Design review of the part shown in the three views and the two pictorial views. Dimensions are in mm from the part's minimum x, y and z. A direction names the side the tool comes from. Coordinates: 2 decimals unless noted, no trailing zeros. Order: outer loops, then holes, each group sorted by start corner. A loop starts at its lowest first (then second) coordinate and runs counter-clockwise, first axis right, second up. Notation, with made-up numbers: (63, -36.75) - (88, -36.75) arc R16 ccw to (88, -31.75) - close; hole circle Ø10 at (23.25, 23.25). An arc over 180 degrees is marked (long way). One line per item, written item: value. Start each with the question number.
(1) To check wall thickness, follow line 1 along Z through (x, y) = (105.5, 37.5); line 2 along X through (y, z) = (26.5, 12); line 3 along Z through (x, y) = (164, 74). State the ranges of each line that lie inside material, in increasing order.
(2) For the marked faces 4, 5, 6 and 7, list the 3-axis set-ups (+Z, -Z, +X, -X, +Y, -Y) from which the entire face can be reached by the end or side of a thin tool; tool diameter is ignored.
(3) Consider section D-D on z = 45.5. Write out the cut boundary in (x, y), then the cut area to 3 significant figures.
(4) Clearance check with flat-ended pins moving along their axes: pin 1 (9.5 mm diameter, centred on x = 22, y = 21.5, fed in from -Z); pin 2 (14 mm diameter, centred on y = 51.5, z = 7.5, fed in from -X); pin 3 (7.5 mm diameter, centred on x = 102, z = 94.5, fed in from -Y). State where each tip first meets the part, or that it passes through.
(5) Consider section A-A on x = 174.5. Write out the cut boundary in (y, z), then the cut area to 3 significant figures.
(6) Consider section C-C on z = 19.5. Write out the cut boundary in (x, y), then the cut area to 3 significant figures.
(7) Mouldability with a two-part tool opening along Z and no side actions: class the marked faces 1, 2 and 3 as released by +Z, released by -Z, zero draft, split by the parting line, or undercut.
(8) Consider section B-B on y = 25.5. Write out the cut boundary in (x, z), then the cut area to 3 significant figures.
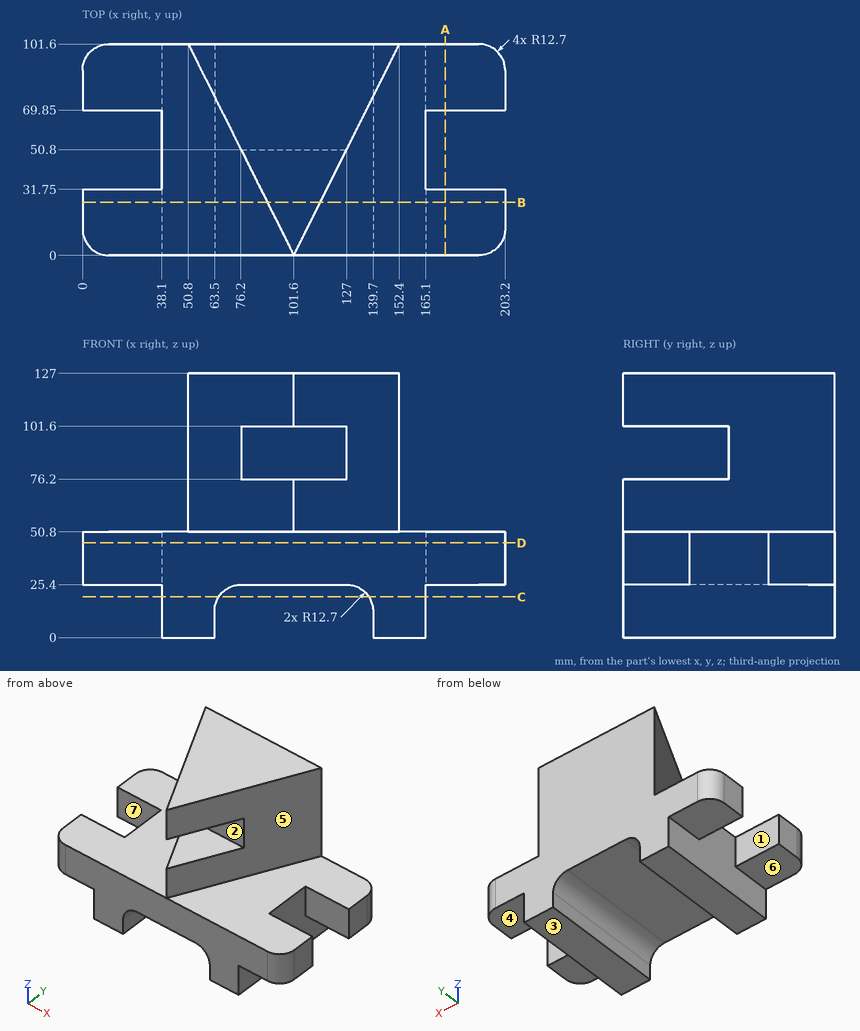
Geometry check:
1. line 1: z = 25.4 to 76.2, 101.6 to 127
1. line 2: x = 38.1 to 63.5, 139.7 to 165.1
1. line 3: z = 0 to 50.8
2. face 4: -Z, +X, +Y, -Y
2. face 5: +Z, +X, -Y
2. face 6: -Z, -X, +Y, -Y
2. face 7: +Z, -Z, -X
3. outline: (0, 12.7) arc R12.7 ccw to (12.7, 0) - (190.5, 0) arc R12.7 ccw to (203.2, 12.7) - (203.2, 31.75) - (165.1, 31.75) - (165.1, 69.85) - (203.2, 69.85) - (203.2, 88.9) arc R12.7 ccw to (190.5, 101.6) - (12.7, 101.6) arc R12.7 ccw to (0, 88.9) - (0, 69.85) - (38.1, 69.85) - (38.1, 31.75) - (0, 31.75) - close
3. area: 17,600 mm^2
4. pin 1: stops at z = 25.4
4. pin 2: stops at x = 38.1
4. pin 3: stops at y = 50.8
5. outline: (0, 25.4) - (31.75, 25.4) - (31.75, 50.8) - (0, 50.8) - close; (69.85, 25.4) - (101.6, 25.4) - (101.6, 50.8) - (69.85, 50.8) - close
5. area: 1,610 mm^2
6. outline: (38.1, 0) - (65.47, 0) - (65.47, 101.6) - (38.1, 101.6) - close; (137.73, 0) - (165.1, 0) - (165.1, 101.6) - (137.73, 101.6) - close
6. area: 5,560 mm^2
7. face 1: zero draft
7. face 2: undercut
7. face 3: released by -Z
8. outline: (0, 25.4) - (38.1, 25.4) - (38.1, 0) - (63.5, 0) - (63.5, 12.7) arc R12.7 cw to (76.2, 25.4) - (127, 25.4) arc R12.7 cw to (139.7, 12.7) - (139.7, 0) - (165.1, 0) - (165.1, 25.4) - (203.2, 25.4) - (203.2, 50.8) - (114.35, 50.8) - (114.35, 76.2) - (88.85, 76.2) - (88.85, 50.8) - (0, 50.8) - close; (88.85, 101.6) - (114.35, 101.6) - (114.35, 127) - (88.85, 127) - close
8. area: 7,820 mm^2
